Part model, mm, in its own coordinate system. A direction names the side the tool comes from. Round coordinates to 2 decimals unless told otherwise and drop trailing zeros. Write each loop counter-clockwise with the first axis right and the second up, starting at its lowest first coordinate (ties: lowest second). Pieces come first, ordered by that corner, then holes. Notation, with made-up numbers: (-15.75, 78) -> (4.25, 78) arc R16 cw to (4.25, 92) -> close; hole circle Ø2 at (35.5, 82). An arc over 180 degrees is marked (long way). Return JSON: item names as keys, results as strings. Group by question number.
(1) Mould opens along Y. For faces 1 (the flat face through (-1, 2, 5)), 2 (the cylindrical face through (-1.874, 43.354, 2.465)), 3 (the flat face through (143.23, -62.05, 2.46)) say: +Y half, -Y half, draft (parallel to the pull), parting line (faces both ways), or undercut.
(2) Tool access for faces 4 (the flat face through (64.72, -55.16, 2.46)), 5 (the flat face through (3, 2, 0)): list every direction of +Z, -Z, +X, -X, +Y, -Y with a clear straight run to the whole face (end or side of a thin tool).
(3) Saw through at A-A (x = 46). List the corners of the cut face in (y, z).
(4) Drill centre lines: L1, parallel to X at y = 8, z = 1.5; L2, parallel to Y at x = -92, z = 1.45; L3, parallel to Y at x = 107, z = 3.85. Where is each one in solid material? Low to high. Write a range as from..to.
(5) Saw through at B-B (z = 4.2). State how many separate pieces and enclosed holes the cut face has, plus the area to 3 significant figures.
(6) Drop flat-ended pins along their axis: pin 1 Ø1.5 at (x, z) = (23, 3) entering from -Y; pin 2 Ø2.5 at (x, z) = (-98.5, 3.5) entering from -Y; pin 3 Ø2.5 at (x, z) = (125.5, 3) entering from +Y; pin 4 Ø2.5 at (x, y) = (-36.16, 26.88) entering from +Z. Give the stop position or say it passes through.
from build123d import *

# Parameters (mm, degrees)
SKETCH1_R           = 12.5
SKETCH1_W           = 33
SKETCH1_H           = 80
BOSS_EXTRUDE1_DEPTH = 5
SKETCH2_R           = 1.6
CUT_EXTRUDE1_DEPTH  = 6
SKETCH4_W           = 5
SKETCH4_H           = 80
CUT_EXTRUDE3_DEPTH  = 6
SKETCH5_R           = 2
CUT_EXTRUDE4_DEPTH  = 6
SKETCH6_R           = 2.5
CUT_EXTRUDE5_DEPTH  = 6
CUT_EXTRUDE7_DEPTH  = 6
SKETCH10_W          = 19.1
SKETCH10_H          = 5
SKETCH10_W_2        = 48.4
CUT_EXTRUDE9_DEPTH  = 6
BOSS_EXTRUDE3_DEPTH = 5
SKETCH12_R          = 2.1
CUT_EXTRUDE10_DEPTH = 5
SKETCH13_R          = 2.1
CUT_EXTRUDE11_DEPTH = 5
SKETCH15_R          = 1.6
BOSS_EXTRUDE4_DEPTH = 5
SKETCH17_R          = 2.1
CUT_EXTRUDE13_DEPTH = 6


with BuildPart() as part:
    # Sketch1 → Boss-Extrude1 (new body)
    with BuildSketch(Plane.XY):
        Polygon((84.001602477, -74.443096951), (130.835354573, -74.443096951), (150.835354573, -54.443096951), (150.835354573, 55.556903049), (130.835354573, 75.556903049), (-129.164645427, 75.556903049), (-149.164645427, 55.556903049), (-149.164645427, -54.443096951), (-129.164645427, -74.443096951), (-82.33089333, -74.443096951), (-49.164645427, -41.276849047), (50.835354573, -41.276849047), align=None)
        with Locations((107.418478525, -54.443096951)):
            Circle(SKETCH1_R, mode=Mode.SUBTRACT)
        with Locations((-105.747769378, -54.443096951)):
            Circle(SKETCH1_R, mode=Mode.SUBTRACT)
        with Locations((0.835354573, 55.556903049)):
            Circle(SKETCH1_R, mode=Mode.SUBTRACT)
        with Locations((89.335354573, 7.157769786)):
            Rectangle(SKETCH1_W, SKETCH1_H, mode=Mode.SUBTRACT)
        with Locations((-87.664645427, 7.157769786)):
            Rectangle(SKETCH1_W, SKETCH1_H, mode=Mode.SUBTRACT)
    extrude(amount=BOSS_EXTRUDE1_DEPTH)

    # Sketch2 → Cut-Extrude1 (cut, through all)
    with BuildSketch(Plane.XY.offset(5)):
        with Locations((17.335354573, -3.276849047)):
            Circle(SKETCH2_R)
        with Locations((17.335354573, -37.276849047)):
            Circle(SKETCH2_R)
        with Locations((-16.664645427, -37.276849047)):
            Circle(SKETCH2_R)
        with Locations((-16.664645427, -3.276849047)):
            Circle(SKETCH2_R)
    extrude(amount=-CUT_EXTRUDE1_DEPTH, mode=Mode.SUBTRACT)

    # Sketch4 → Cut-Extrude3 (cut, through all)
    with BuildSketch(Plane.XY.offset(5)):
        with Locations((148.335354573, 7.157769786)):
            Rectangle(SKETCH4_W, SKETCH4_H)
        with Locations((-146.664645427, 7.157769786)):
            Rectangle(SKETCH4_W, SKETCH4_H)
    extrude(amount=-CUT_EXTRUDE3_DEPTH, mode=Mode.SUBTRACT)

    # Sketch5 → Cut-Extrude4 (cut, through all)
    with BuildSketch(Plane.XY.offset(5)):
        with Locations((-67.164645427, -8.117475471)):
            Circle(SKETCH5_R)
        with Locations((-36.164645427, -8.117475471)):
            Circle(SKETCH5_R)
        with Locations((-36.164645427, 26.882524529)):
            Circle(SKETCH5_R)
        with Locations((-67.164645427, 26.882524529)):
            Circle(SKETCH5_R)
        with Locations((68.835354573, 26.882524529)):
            Circle(SKETCH5_R)
        with Locations((37.835354573, 26.882524529)):
            Circle(SKETCH5_R)
        with Locations((37.835354573, -8.117475471)):
            Circle(SKETCH5_R)
        with Locations((68.835354573, -8.117475471)):
            Circle(SKETCH5_R)
    extrude(amount=-CUT_EXTRUDE4_DEPTH, mode=Mode.SUBTRACT)

    # Sketch6 → Cut-Extrude5 (cut, through all)
    with BuildSketch(Plane.XY.offset(5)):
        with Locations((133.835354573, -18.342230214)):
            Circle(SKETCH6_R)
        with Locations((133.835354573, 32.657769786)):
            Circle(SKETCH6_R)
        with Locations((-132.164645427, 32.657769786)):
            Circle(SKETCH6_R)
        with Locations((-132.164645427, -18.342230214)):
            Circle(SKETCH6_R)
    extrude(amount=-CUT_EXTRUDE5_DEPTH, mode=Mode.SUBTRACT)

    # Sketch7 → Cut-Extrude7 (cut, through all)
    with BuildSketch(Plane.XY.offset(5)):
        Polygon((-115.747769378, -69.443096951), (-134.164645427, -69.443096951), (-129.164645427, -74.443096951), (-115.747769378, -74.443096951), align=None)
        Polygon((-95.747769378, -74.443096951), (-95.747769378, -69.443096951), (-77.33089333, -69.443096951), (-82.33089333, -74.443096951), align=None)
        Polygon((97.418478525, -74.443096951), (84.001602477, -74.443096951), (79.001602477, -69.443096951), (97.418478525, -69.443096951), align=None)
        Polygon((130.835354573, -74.443096951), (117.418478525, -74.443096951), (117.418478525, -69.443096951), (135.835354573, -69.443096951), align=None)
    extrude(amount=-CUT_EXTRUDE7_DEPTH, mode=Mode.SUBTRACT)

    # Sketch10 → Cut-Extrude9 (cut, through all)
    with BuildSketch(Plane.XY.offset(5)):
        with Locations((-111.214645427, 73.056903049)):
            Rectangle(SKETCH10_W, SKETCH10_H)
        with Locations((-72.114645427, 73.056903049)):
            Rectangle(SKETCH10_W, SKETCH10_H)
        with Locations((-38.364645427, 73.056903049)):
            Rectangle(SKETCH10_W_2, SKETCH10_H)
        Polygon((83.335354573, 75.556903049), (83.335354573, 70.556903049), (64.235354573, 70.556903049), (15.835354573, 70.556903049), (15.835354573, 75.556903049), (64.235354573, 75.556903049), align=None)
        with Locations((112.885354573, 73.056903049)):
            Rectangle(SKETCH10_W, SKETCH10_H)
    extrude(amount=-CUT_EXTRUDE9_DEPTH, mode=Mode.SUBTRACT)

    # Sketch11 → Boss-Extrude3 (add)
    with BuildSketch(Plane.XY.offset(5)):
        with BuildLine():
            Line((103.088351506, -74.443096951), (111.748605544, -74.443096951))
            ThreePointArc((111.748605544, -74.443096951), (107.418478525, -76.943096951), (103.088351506, -74.443096951))
        make_face()
        with BuildLine():
            Line((-110.077896397, -74.443096951), (-101.417642359, -74.443096951))
            ThreePointArc((-101.417642359, -74.443096951), (-105.747769378, -76.943096951), (-110.077896397, -74.443096951))
        make_face()
        with BuildLine():
            Line((97.665481592, 75.556903049), (89.005227555, 75.556903049))
            ThreePointArc((89.005227555, 75.556903049), (93.335354573, 78.056903049), (97.665481592, 75.556903049))
        make_face()
        with BuildLine():
            Line((5.165481592, 75.556903049), (-3.494772445, 75.556903049))
            ThreePointArc((-3.494772445, 75.556903049), (0.835354573, 78.056903049), (5.165481592, 75.556903049))
        make_face()
        with BuildLine():
            Line((-87.334518408, 75.556903049), (-95.994772445, 75.556903049))
            ThreePointArc((-95.994772445, 75.556903049), (-91.664645427, 78.056903049), (-87.334518408, 75.556903049))
        make_face()
    extrude(amount=-BOSS_EXTRUDE3_DEPTH)

    # Sketch12 → Cut-Extrude10 (cut)
    with BuildSketch(Plane.XY.offset(5)):
        with Locations((107.418478525, -71.943096951)):
            Circle(SKETCH12_R)
        with Locations((-105.747769378, -71.943096951)):
            Circle(SKETCH12_R)
        with Locations((93.335354573, 73.056903049)):
            Circle(SKETCH12_R)
        with Locations((0.835354573, 73.056903049)):
            Circle(SKETCH12_R)
        with Locations((-91.664645427, 73.056903049)):
            Circle(SKETCH12_R)
    extrude(amount=-CUT_EXTRUDE10_DEPTH, mode=Mode.SUBTRACT)

    # Sketch13 → Cut-Extrude11 (cut)
    with BuildSketch(Plane.XY.offset(5)):
        with Locations((-19.664645427, 55.556903049)):
            Circle(SKETCH13_R)
        with Locations((21.335354573, 55.556903049)):
            Circle(SKETCH13_R)
        with Locations((-126.247769378, -54.443096951)):
            Circle(SKETCH13_R)
        with Locations((-85.247769378, -54.443096951)):
            Circle(SKETCH13_R)
        with Locations((86.918478525, -54.443096951)):
            Circle(SKETCH13_R)
        with Locations((127.918478525, -54.443096951)):
            Circle(SKETCH13_R)
    extrude(amount=-CUT_EXTRUDE11_DEPTH, mode=Mode.SUBTRACT)

    # Sketch15 → Boss-Extrude4 (add)
    with BuildSketch(Plane(origin=(0, 0, 0), x_dir=(-1, 0, 0), z_dir=(0, 0, -1))):
        with Locations((16.664645427, -37.276849047)):
            Circle(SKETCH15_R)
        with Locations((16.664645427, -3.276849047)):
            Circle(SKETCH15_R)
        with Locations((-17.335354573, -37.276849047)):
            Circle(SKETCH15_R)
        with Locations((-17.335354573, -3.276849047)):
            Circle(SKETCH15_R)
    extrude(amount=-BOSS_EXTRUDE4_DEPTH)

    # Sketch17 → Cut-Extrude13 (cut, through all)
    with BuildSketch(Plane.XY.offset(5)):
        with Locations((-16.164645427, 1.723150953)):
            Circle(SKETCH17_R)
        with Locations((17.835354573, 1.723150953)):
            Circle(SKETCH17_R)
        with Locations((17.835354573, -32.276849047)):
            Circle(SKETCH17_R)
        with Locations((-16.164645427, -32.276849047)):
            Circle(SKETCH17_R)
    extrude(amount=-CUT_EXTRUDE13_DEPTH, mode=Mode.SUBTRACT)


solid = part.part
Computed values:
{
 "1": {"face 1": "draft", "face 2": "undercut", "face 3": "-Y half"},
 "2": {"face 4": "+Z, -Z, -Y", "face 5": "-Z, +X, -X, +Y, -Y"},
 "3": {"outline": "(-41.28, 0) -> (70.56, 0) -> (70.56, 5) -> (-41.28, 5) -> close"},
 "4": {"L1": "-144.16..-104.16, -71.16..72.84, 105.84..145.84", "L2": "-69.44..-32.84, 47.16..70.98, 75.13..78.05", "L3": "-76.93..-74, -69.89..-66.94, -41.95..70.56"},
 "5": {"separate pieces": "1", "enclosed holes": "32", "area": "30,700 mm2"},
 "6": {"pin 1": "y = -41.28", "pin 2": "y = -74.44", "pin 3": "y = 75.56", "pin 4": "through"}
}
